Geometry check sheet. Reference: the model listing, model coordinates, mm. A direction names the side the tool comes from. Coordinates: 2 decimals unless noted, no trailing zeros. Write each loop counter-clockwise with the first axis right and the second up, starting at its lowest first coordinate (ties: lowest second). Pieces come first, ordered by that corner, then holes. Notation, with made-up numbers: (22, 85) -> (73, 85) arc R27 cw to (73, 112) -> close; hole circle Ø9 at (12.5, -16.75). An arc over 180 degrees is marked (long way). Use a Markdown table: item, result.
```python
from build123d import *

# Parameters (mm, degrees)
F0_W     = 100
F0_H     = 70
F1_DEPTH = 45
F2_T     = -5
F4_DEPTH = 40
F6_D     = 5.5
F7_R     = 10.5
F8_DEPTH = 100.001
F10_R    = 5


with BuildPart() as f1:
    # F0 (on Top) → F1 (new body)
    with BuildSketch(Plane.XY):
        with Locations((-0.4376240075, -0.4940965772)):
            Rectangle(F0_W, F0_H)
    extrude(amount=F1_DEPTH)

    # F2
    f2_openings = [f1.faces().sort_by_distance(p)[0] for p in [
        (-0.437624, -0.494097, 45),
    ]]
    offset(amount=F2_T, openings=f2_openings)

    # F3 (on face) → F4 (join, through all)
    with BuildSketch(Plane.XY.offset(5)):
        with BuildLine():
            ThreePointArc((-45.4376240075, 22.0059034228), (-40.1343231486, 24.2026025639), (-37.9376240075, 29.5059034228))
            Line((-37.9376240075, 29.5059034228), (-45.4376240075, 29.5059034228))
            Line((-45.4376240075, 29.5059034228), (-45.4376240075, 22.0059034228))
        make_face()
        with BuildLine():
            ThreePointArc((-37.9376240075, -30.4940965772), (-40.1343231486, -25.1907957183), (-45.4376240075, -22.9940965772))
            Line((-45.4376240075, -22.9940965772), (-45.4376240075, -30.4940965772))
            Line((-45.4376240075, -30.4940965772), (-37.9376240075, -30.4940965772))
        make_face()
        with BuildLine():
            Line((44.5623759925, 29.5059034228), (37.0623759925, 29.5059034228))
            ThreePointArc((37.0623759925, 29.5059034228), (39.2590751336, 24.2026025639), (44.5623759925, 22.0059034228))
            Line((44.5623759925, 22.0059034228), (44.5623759925, 29.5059034228))
        make_face()
        with BuildLine():
            Line((44.5623759925, -30.4940965772), (44.5623759925, -22.9940965772))
            ThreePointArc((44.5623759925, -22.9940965772), (39.2590751336, -25.1907957183), (37.0623759925, -30.4940965772))
            Line((37.0623759925, -30.4940965772), (44.5623759925, -30.4940965772))
        make_face()
    extrude(amount=F4_DEPTH)

    # F6 (through all)
    with Locations(Plane.XY.offset(45)):
        with Locations((44.5623759925, 29.5059034228), (44.5623759925, -30.4940965772), (-45.4376240075, -30.4940965772), (-45.4376240075, 29.5059034228)):
            Hole(F6_D / 2)

    # F7 (on face) → F8 (cut, through all)
    with BuildSketch(Plane(origin=(-50.4376240075, 0, 0), x_dir=(0, -1, 0), z_dir=(-1, 0, 0))):
        with Locations((0.4940965772, 22.5)):
            Circle(F7_R)
    extrude(amount=-F8_DEPTH, mode=Mode.SUBTRACT)

    # F10
    f10_edges = [f1.edges().sort_by_distance(p)[0] for p in [
        (-50.437624, 34.505903, 22.5),
        (49.562376, 34.505903, 22.5),
        (-50.437624, -35.494097, 22.5),
        (49.562376, -35.494097, 22.5),
    ]]
    fillet(f10_edges, radius=F10_R)


solid = f1.part
```
Item 1: Mould release check, pull along Z, two halves, no side actions. Record for faces 1 (the cylindrical face through (47.027, -6.139, 31.354)), 2 (the cylindrical face through (39.32, -25.13, 24.72)), 3 (the flat face through (-1, -31, 45)): +Z half, -Z half, draft (parallel to the pull), parting line (faces both ways), or undercut.
Answer block:
| item | result |
|---|---|
| face 1 | undercut |
| face 2 | draft |
| face 3 | +Z half |
Item 2: Section check A-A on z = 22.5. Record the boundary of the cut face in (x, y).
Answer block:
| item | result |
|---|---|
| outline | (-50.44, -30.49) arc R5 ccw to (-45.44, -35.49) -> (44.56, -35.49) arc R5 ccw to (49.56, -30.49) -> (49.56, -10.99) -> (44.56, -10.99) -> (44.56, -22.99) arc R7.5 ccw to (37.06, -30.49) -> (-37.94, -30.49) arc R7.5 ccw to (-45.44, -22.99) -> (-45.44, -10.99) -> (-50.44, -10.99) -> close; (-50.44, 10.01) -> (-45.44, 10.01) -> (-45.44, 22.01) arc R7.5 ccw to (-37.94, 29.51) -> (37.06, 29.51) arc R7.5 ccw to (44.56, 22.01) -> (44.56, 10.01) -> (49.56, 10.01) -> (49.56, 29.51) arc R5 ccw to (44.56, 34.51) -> (-45.44, 34.51) arc R5 ccw to (-50.44, 29.51) -> close; hole circle Ø5.5 at (-45.44, -30.49); hole circle Ø5.5 at (-45.44, 29.51); hole circle Ø5.5 at (44.56, -30.49); hole circle Ø5.5 at (44.56, 29.51) |
Item 3: Section check C-C on x = -23.5. Record the boundary of the cut face in (y, z).
Answer block:
| item | result |
|---|---|
| outline | (-35.49, 0) -> (34.51, 0) -> (34.51, 45) -> (29.51, 45) -> (29.51, 5) -> (-30.49, 5) -> (-30.49, 45) -> (-35.49, 45) -> close |
Item 4: Section check D-D on y = -25.5. Record the boundary of the cut face in (x, z), then the cut area to 3 significant figures.
Answer block:
| item | result |
|---|---|
| outline | (-50.44, 0) -> (49.56, 0) -> (49.56, 45) -> (38.97, 45) -> (38.97, 5) -> (-39.84, 5) -> (-39.84, 45) -> (-50.44, 45) -> close |
| area | 1,350 mm^2 |
Item 5: Depth check by flat-ended pin: P1, Ø18, axis at x = 7.5, y = -5.5, coming from the +Z side; P2, Ø19, axis at y = -0.49, z = 22.5, coming from the -X side. Enter the tip coordinate at first touch or a pass-through.
Answer block:
| item | result |
|---|---|
| P1 | stops at z = 5 |
| P2 | passes through |
Item 6: Tool access check on faces 4 (the cylindrical face through (-47.973, -6.139, 31.354)), 5 (the cylindrical face through (39.2, 24.26, 24.72)). Record the directions out of +Z, -Z, +X, -X, +Y, -Y that give a thin tool (end or side, any length) a straight path to the whole face; none if there is none.
Answer block:
| item | result |
|---|---|
| face 4 | +X, -X |
| face 5 | +Z |
Item 7: Thickness scan on L1, parallel to X at y = -28, z = 27; L2, parallel to X at y = 16, z = 23; L3, parallel to Y at x = -31, z = 42. Record the ranges inside material, lowest first. Write a range as [from, to].
Answer block:
| item | result |
|---|---|
| L1 | x = [-50.44, -46.6], [-44.28, -38.36], [37.49, 43.4], [45.72, 49.56] |
| L2 | x = [-50.44, -45.44], [44.56, 49.56] |
| L3 | y = [-35.49, -30.49], [29.51, 34.51] |
Item 8: Section check B-B on z = 40. Record the boundary of the cut face in (x, y), then the cut area to 3 significant figures.
Answer block:
| item | result |
|---|---|
| outline | (-50.44, -30.49) arc R5 ccw to (-45.44, -35.49) -> (44.56, -35.49) arc R5 ccw to (49.56, -30.49) -> (49.56, 29.51) arc R5 ccw to (44.56, 34.51) -> (-45.44, 34.51) arc R5 ccw to (-50.44, 29.51) -> close; hole circle Ø5.5 at (-45.44, -30.49); hole circle Ø5.5 at (-45.44, 29.51); hole (-45.44, -22.99) arc R7.5 cw to (-37.94, -30.49) -> (37.06, -30.49) arc R7.5 cw to (44.56, -22.99) -> (44.56, 22.01) arc R7.5 cw to (37.06, 29.51) -> (-37.94, 29.51) arc R7.5 cw to (-45.44, 22.01) -> close; hole circle Ø5.5 at (44.56, -30.49); hole circle Ø5.5 at (44.56, 29.51) |
| area | 1,660 mm^2 |
